from build123d import *
from build123d.topology import SkipClean

# Parameters (mm, degrees)
BOSS_EXTRU_1_DEPTH           = 5
BOSS_EXTRU_2_DEPTH           = 15
ESQUISSE3_R                  = 1.6
ENL_V_MAT_EXTRU_1_DEPTH      = 70.166465863
ESQUISSE4_R                  = 2.9
ESQUISSE4_R_2                = 1.6
ENL_V_MAT_EXTRU_2_DEPTH      = 26
ENL_V_MAT_EXTRU_2_DEPTH_BACK = 26
ENL_V_MAT_EXTRU_3_DEPTH      = 25
ESQUISSE6_R                  = 2.9
ESQUISSE6_R_2                = 1.6
ENL_V_MAT_EXTRU_4_DEPTH      = 25
ENL_V_MAT_EXTRU_4_DEPTH_BACK = 10


with BuildPart() as part:
    # Esquisse1 → Boss.-Extru.1 (new body)
    with BuildSketch(Plane.XY):
        Polygon((15, 15), (2, 28), (0, 28), (0, 0), (20, 0), (20, -2.9), (39.8, -2.9), (39.8, 0), (60, 0), (60, 28), (58, 28), (45, 15), align=None)
    extrude(amount=BOSS_EXTRU_1_DEPTH)

    # Esquisse2 → Boss.-Extru.2 (add)
    with BuildSketch(Plane.XY.offset(5)):
        with BuildLine():
            Line((2, 28), (0, 28))
            Line((0, 28), (0, 0))
            Line((0, 0), (20, 0))
            Line((20, 0), (20, -2.9))
            Line((20, -2.9), (24.9, -2.9))
            ThreePointArc((24.9, -2.9), (29.9, 2.1), (34.9, -2.9))
            Line((34.9, -2.9), (39.8, -2.9))
            Line((39.8, -2.9), (39.8, 0))
            Line((39.8, 0), (60, 0))
            Line((60, 0), (60, 28))
            Line((60, 28), (58, 28))
            Line((58, 28), (45, 15))
            Line((45, 15), (15, 15))
            Line((15, 15), (2, 28))
        make_face()
    extrude(amount=BOSS_EXTRU_2_DEPTH)

    # Esquisse3 → Enl_v. mat.-Extru.1 (cut, through all)
    with BuildSketch(Plane(origin=(60, 0, 0), x_dir=(0, 0, -1), z_dir=(1, 0, 0))):
        with Locations((-10, 20)):
            Circle(ESQUISSE3_R)
    extrude(amount=-ENL_V_MAT_EXTRU_1_DEPTH, mode=Mode.SUBTRACT)

    # Esquisse4 → Enl_v. mat.-Extru.2 (cut, two sides)
    with BuildSketch(Plane.ZY.offset(-30)) as enl_v_mat_extru_2_sk:
        with Locations(Location((10, 20, 0), (0, 0, 90))):
            Circle(ESQUISSE4_R)
        with Locations(Location((10, 20, 0), (0, 0, 180))):
            Circle(ESQUISSE4_R_2, mode=Mode.SUBTRACT)
    extrude(amount=ENL_V_MAT_EXTRU_2_DEPTH, mode=Mode.SUBTRACT)
    extrude(enl_v_mat_extru_2_sk.sketch, amount=-ENL_V_MAT_EXTRU_2_DEPTH_BACK, mode=Mode.SUBTRACT)

    # Esquisse5 → Enl_v. mat.-Extru.3 (cut)
    with BuildSketch(Plane.XZ):
        with BuildLine():
            ThreePointArc((8.86862915, 11.13137085), (8.86862915, 8.86862915), (11.13137085, 8.86862915))
            Line((11.13137085, 8.86862915), (8.86862915, 11.13137085))
        make_face()
        with BuildLine():
            Line((8.86862915, 11.13137085), (11.13137085, 8.86862915))
            ThreePointArc((11.13137085, 8.86862915), (11.478207252, 9.387706508), (11.6, 10))
            ThreePointArc((11.6, 10), (10.612293492, 11.478207252), (8.86862915, 11.13137085))
        make_face()
        with BuildLine():
            ThreePointArc((51.036985489, 11.125728207), (48.774271793, 11.136985489), (48.763014511, 8.874271793))
            Line((48.763014511, 8.874271793), (51.036985489, 11.125728207))
        make_face()
        with BuildLine():
            Line((51.036985489, 11.125728207), (48.763014511, 8.874271793))
            ThreePointArc((48.763014511, 8.874271793), (50.508614499, 8.520274217), (51.5, 10))
            ThreePointArc((51.5, 10), (51.379725783, 10.608614499), (51.036985489, 11.125728207))
        make_face()
    extrude(amount=-ENL_V_MAT_EXTRU_3_DEPTH, mode=Mode.SUBTRACT)

    # Esquisse6 → Enl_v. mat.-Extru.4 (cut, two sides)
    with SkipClean():  # the faces are left unmerged after this step: merging them gives an invalid solid
        with BuildSketch(Plane(origin=(0, 15, 0), x_dir=(1, 0, 0), z_dir=(0, 1, 0))) as enl_v_mat_extru_4_sk:
            with Locations(Location((10, -10, 0), (0, 0, 270))):
                Circle(ESQUISSE6_R)
            with Locations(Location((10, -10, 0), (0, 0, 90))):
                Circle(ESQUISSE6_R_2, mode=Mode.SUBTRACT)
            with Locations(Location((49.9, -10, 0), (0, 0, 89.012092783))):
                Circle(ESQUISSE6_R)
            with Locations(Location((49.9, -10, 0), (0, 0, 90))):
                Circle(ESQUISSE6_R_2, mode=Mode.SUBTRACT)
        extrude(amount=ENL_V_MAT_EXTRU_4_DEPTH, mode=Mode.SUBTRACT)
        extrude(enl_v_mat_extru_4_sk.sketch, amount=-ENL_V_MAT_EXTRU_4_DEPTH_BACK, mode=Mode.SUBTRACT)


solid = part.part
Could you check a few things on this model? Use its own coordinates, in mm. A direction names the side the tool comes from. Give positions to 0.01 mm unless a question says otherwise; leave off trailing zeros. Loops run counter-clockwise (first coordinate to the right, second up) from the corner with the lowest first, then second, coordinate; pieces in that order, holes last. Notation, with made-up numbers: (-7, 85.25) -> (26, 85.25) arc R19 ccw to (26, 107.25) -> close; hole circle Ø11 at (-30.75, -16). An arc over 180 degrees is marked (long way). Return JSON: item names as keys, results as strings.
Item 1: We'd pull the mould along X, two halves only. Please class faces 1 (the flat face through (53, 23, 8)), 2 (the flat face through (39.8, -1, 10)), 3 (the flat face through (30, -2.9, 3)): +X half, -X half, draft (parallel to the pull), parting line (faces both ways), or undercut.
Geometry results:
{"face 1": "undercut", "face 2": "+X half", "face 3": "draft"}
Item 2: I'm going to push flat-ended pins straight in: pin 1 (8 mm diameter, centred on x = 47, z = 15.5, fed in from +Y); pin 2 (1 mm diameter, centred on x = 6.5, z = 8, fed in from +Y); pin 3 (3 mm diameter, centred on x = 10, z = 9.5, fed in from +Y). Where does each tip first touch, or does it pass through?
Geometry results:
{"pin 1": "stops at y = 21", "pin 2": "stops at y = 24", "pin 3": "stops at y = 5"}
Item 3: I need wall thicknesses on L1, parallel to X at y = 9, z = 10; L2, parallel to Z at x = 2, y = 20; L3, parallel to X at y = 17.9, z = 10. Which ranges of each line are inside material? Lowest first, please. Write a range as from..to.
Geometry results:
{"L1": "x = 0..7.1, 12.9..47, 52.8..60", "L2": "z = 0..8.4, 11.6..20", "L3": "x = 0..4, 56..60"}
Item 4: If we section it at B-B on x = 55: List the corners of the cut face in (y, z) for me, plus the area to 3 significant figures.
Geometry results:
{"outline": "(0, 0) -> (25, 0) -> (25, 20) -> (0, 20) -> close; hole circle Ø5.8 at (20, 10)", "area": "474 mm²"}
Item 5: Which directions (+Z, -Z, +X, -X, +Y, -Y) give clear straight access to the entire face, cutting with the end or side of a thin tool? Please do faces 4 (the cylindrical face through (6.375, 21.559, 7.555)), 5 (the flat face through (51.2, 5, 8.8)), 6 (the flat face through (30, 15, 10)).
Geometry results:
{"face 4": "none", "face 5": "+Y", "face 6": "+Z, -Z, +Y"}
Item 6: If we section it at D-D on x = 29.9: List the corners of the cut face in (y, z) for me, plus the area to 3 significant figures.
Geometry results:
{"outline": "(-2.9, 0) -> (15, 0) -> (15, 20) -> (2.1, 20) -> (2.1, 5) -> (-2.9, 5) -> close", "area": "283 mm²"}
Item 7: If we section it at C-C on z = 17.5: List the corners of the cut face in (x, y) for me.
Geometry results:
{"outline": "(0, 0) -> (20, 0) -> (20, -2.9) -> (24.9, -2.9) arc R5 cw to (34.9, -2.9) -> (39.8, -2.9) -> (39.8, 0) -> (60, 0) -> (60, 28) -> (58, 28) -> (45, 15) -> (15, 15) -> (2, 28) -> (0, 28) -> close"}
Item 8: If we section it at A-A on y = 23.5: List the corners of the cut face in (x, z) for me.
Geometry results:
{"outline": "(0, 0) -> (6.5, 0) -> (6.5, 20) -> (0, 20) -> close; (53.5, 0) -> (60, 0) -> (60, 20) -> (53.5, 20) -> close"}
